```python
from build123d import *

# Parameters (mm, degrees)
SKETCH1_R           = 9.906
BOSS_EXTRUDE1_DEPTH = 508
CUT_EXTRUDE1_START  = 20.32
SKETCH2_R           = 3.175
CUT_EXTRUDE1_DEPTH  = 22.86
SCALE1_SCALE        = 0.25


with BuildPart() as part:
    # Sketch1 → Boss-Extrude1 (new body)
    with BuildSketch(Plane(origin=(0, 0, 0), x_dir=(1, 0, 0), z_dir=(0, 1, 0))):
        with Locations(Location((0, 0, 0), (0, 0, 270))):
            Circle(SKETCH1_R)
    extrude(amount=BOSS_EXTRUDE1_DEPTH)

    # Sketch2 → Cut-Extrude1 (cut)
    with BuildSketch(Plane(origin=(0, 0, 0), x_dir=(0, 0, -1), z_dir=(1, 0, 0)).offset(CUT_EXTRUDE1_START)):
        with Locations((0, 498.602)):
            Circle(SKETCH2_R)
    cut_extrude1 = extrude(amount=-CUT_EXTRUDE1_DEPTH, mode=Mode.SUBTRACT)

    # Mirror1: Cut-Extrude1 across plane
    add(cut_extrude1.mirror(Plane.ZX.offset(254)), mode=Mode.SUBTRACT)


with BuildPart() as part_1:
    # Scale1: scaled about (-0.018116733, 254, 1.117e-06)
    add(part.part.scale(SCALE1_SCALE).moved(Location((-0.01358755, 190.5, 8.38e-07))))


solid = part_1.part
```
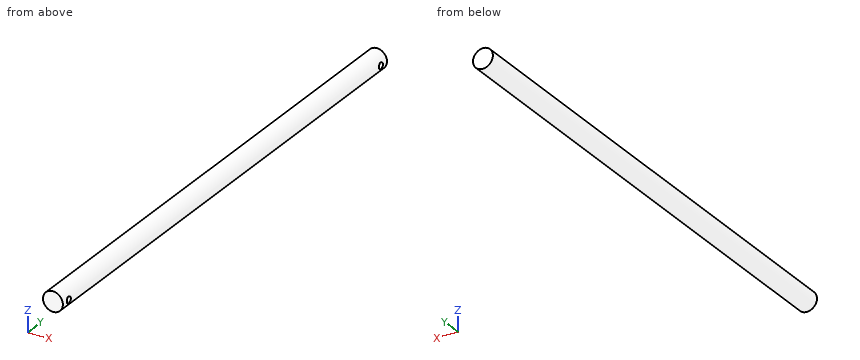
The listing builds one solid part. Answer for the finished solid, in the listing's coordinates (mm). Round coordinates to 2 decimals unless told otherwise and drop trailing zeros. Loops run counter-clockwise (first coordinate to the right, second up) from the corner with the lowest first, then second, coordinate; pieces in that order, holes last.
Q1. Given pin 1 Ø2 at (y, z) = (214, 1.5) entering from +X; pin 2 Ø1.3 at (y, z) = (315.5, 0) entering from +X, each flat-ended and moving along its own axis, determine where each tip first touches the part or whether it passes through.
Q2. Section B-B, the plane x = 1.05 is taken. Determine the outline of the cut face in (y, z), then the cut area to 3 significant figures.
Q3. Section A-A, the plane z = 0 is taken. Determine the outline of the cut face in (x, y), then the cut area to 3 significant figures.
Q4. Find the intervals of material crossed by line 1 (Y direction, x = 0.4, z = 0); line 2 (X direction, y = 307, z = -0.35); line 3 (Y direction, x = 1.85, z = -0.7), in increasing order.
Q5. Section C-C, the plane y = 234 is taken. Determine the outline of the cut face in (x, z).
Completed:
1. pin 1: stops at x = 2.41
1. pin 2: stops at x = 2.46
2. outline: (190.5, -2.24) - (317.5, -2.24) - (317.5, 2.24) - (190.5, 2.24) - close; hole circle Ø1.59 at (192.85, 0); hole circle Ø1.59 at (315.15, 0)
2. area: 564 mm2
3. outline: (-2.49, 190.5) - (2.46, 190.5) - (2.46, 192.06) - (-0.65, 192.06) - (-0.65, 193.64) - (2.46, 193.64) - (2.46, 314.36) - (-0.65, 314.36) - (-0.65, 315.94) - (2.46, 315.94) - (2.46, 317.5) - (-2.49, 317.5) - close
3. area: 619 mm2
4. line 1: y = 190.5 to 192.06, 193.64 to 314.36, 315.94 to 317.5
4. line 2: x = -2.47 to 2.44
4. line 3: y = 190.5 to 192.48, 193.22 to 314.78, 315.52 to 317.5
5. outline: circle Ø4.95 at (-0.01, 0)
